Work out the finished part from the listing and answer in its coordinate system (mm). Face numbers are marked on the shaded views. A direction names the side the tool comes from. Coordinates: 2 decimals unless noted, no trailing zeros. Write each loop counter-clockwise with the first axis right and the second up, starting at its lowest first coordinate (ties: lowest second). Pieces come first, ordered by that corner, then holes. Notation, with made-up numbers: (22.5, -2.5) - (81.5, -2.5) arc R17 cw to (81.5, 26.5) - close; hole circle Ø10 at (21, 88). An arc over 180 degrees is marked (long way). One line per item, written item: value.
```python
from build123d import *

# Parameters (mm, degrees)
ESBO_O1_W                                   = 50
ESBO_O1_H                                   = 57
ESBO_O1_R                                   = 13
RESSALTO_EXTRUS_O1_DEPTH                    = 8
ESBO_O3_W                                   = 50
ESBO_O3_H                                   = 57
RESSALTO_EXTRUS_O2_DEPTH                    = 2
BROCA_DE_ROSQUEAR_PARA_TARRAXA_DE_M51_D     = 4.2
BROCA_DE_ROSQUEAR_PARA_TARRAXA_DE_M51_DEPTH = 15
BROCA_DE_ROSQUEAR_PARA_TARRAXA_DE_M51_TIP   = 1.2618073
BROCA_DE_ROSQUEAR_PARA_TARRAXA_DE_M52_D     = 4.2
BROCA_DE_ROSQUEAR_PARA_TARRAXA_DE_M52_DEPTH = 15
BROCA_DE_ROSQUEAR_PARA_TARRAXA_DE_M52_TIP   = 1.2618073


with BuildPart() as part:
    # Esboço1 → Ressalto-extrusão1 (new body)
    with BuildSketch(Plane.XY):
        with Locations((25, 28.5)):
            Rectangle(ESBO_O1_W, ESBO_O1_H)
        with Locations((25, 25)):
            Circle(ESBO_O1_R, mode=Mode.SUBTRACT)
    extrude(amount=RESSALTO_EXTRUS_O1_DEPTH)

    # Esboço3 → Ressalto-extrusão2 (add)
    with BuildSketch(Plane.XY.offset(8)):
        with Locations((25, 28.5)):
            Rectangle(ESBO_O3_W, ESBO_O3_H)
    extrude(amount=RESSALTO_EXTRUS_O2_DEPTH)

    # Broca de rosquear para tarraxa de M51
    with Locations(Plane(origin=(0, 0, 0), x_dir=(-1, 0, 0), z_dir=(0, -1, 0))):
        with Locations((-6, -5), (-44, -5)):
            Hole(BROCA_DE_ROSQUEAR_PARA_TARRAXA_DE_M51_D / 2, depth=BROCA_DE_ROSQUEAR_PARA_TARRAXA_DE_M51_DEPTH)
            with Locations((0, 0, -(BROCA_DE_ROSQUEAR_PARA_TARRAXA_DE_M51_DEPTH + BROCA_DE_ROSQUEAR_PARA_TARRAXA_DE_M51_TIP / 2))):  # 118° drill point
                Cone(0, BROCA_DE_ROSQUEAR_PARA_TARRAXA_DE_M51_D / 2, BROCA_DE_ROSQUEAR_PARA_TARRAXA_DE_M51_TIP, mode=Mode.SUBTRACT)

    # Broca de rosquear para tarraxa de M52
    with Locations(Plane(origin=(0, 57, 0), x_dir=(1, 0, 0), z_dir=(0, 1, 0))):
        with Locations((6, -5), (44, -5)):
            Hole(BROCA_DE_ROSQUEAR_PARA_TARRAXA_DE_M52_D / 2, depth=BROCA_DE_ROSQUEAR_PARA_TARRAXA_DE_M52_DEPTH)
            with Locations((0, 0, -(BROCA_DE_ROSQUEAR_PARA_TARRAXA_DE_M52_DEPTH + BROCA_DE_ROSQUEAR_PARA_TARRAXA_DE_M52_TIP / 2))):  # 118° drill point
                Cone(0, BROCA_DE_ROSQUEAR_PARA_TARRAXA_DE_M52_D / 2, BROCA_DE_ROSQUEAR_PARA_TARRAXA_DE_M52_TIP, mode=Mode.SUBTRACT)


solid = part.part
```
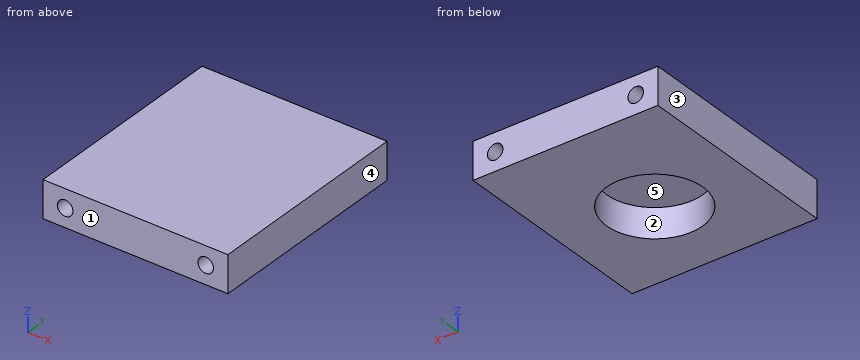
Item 1: Determine the mould class of the marked faces 1, 2 and 3 for opening direction Y: +Y half, -Y half, draft (parallel to the pull), parting line (faces both ways), or undercut.
Evaluation:
face 1: -Y half
face 2: undercut
face 3: draft
Item 2: Section D-D, the plane y = 25 is taken. Determine the outline of the cut face in (x, z), then the cut area to 3 significant figures.
Evaluation:
outline: (0, 0) - (12, 0) - (12, 8) - (38, 8) - (38, 0) - (50, 0) - (50, 10) - (0, 10) - close
area: 292 mm2
Item 3: Section B-B, the plane x = 25 is taken. Determine the outline of the cut face in (y, z).
Evaluation:
outline: (0, 0) - (12, 0) - (12, 8) - (38, 8) - (38, 0) - (57, 0) - (57, 10) - (0, 10) - close
Item 4: Given pin 1 (2.5 mm diameter, centred on x = 6, z = 5, fed in from -Y); pin 2 (4 mm diameter, centred on x = 44, z = 5, fed in from -Y); pin 3 (13 mm diameter, centred on x = 22.5, y = 26, fed in from -Z), each flat-ended and moving along its own axis, determine where each tip first touches the part or whether it passes through.
Evaluation:
pin 1: stops at y = 15.51
pin 2: stops at y = 15.06
pin 3: stops at z = 8
Item 5: Section A-A, the plane z = 1.25 is taken. Determine the outline of the cut face in (x, y).
Evaluation:
outline: (0, 0) - (50, 0) - (50, 57) - (0, 57) - close; hole circle Ø26 at (25, 25)
Item 6: Section C-C, the plane y = 11 is taken. Determine the outline of the cut face in (x, z).
Evaluation:
outline: (0, 0) - (50, 0) - (50, 10) - (0, 10) - close; hole circle Ø4.2 at (6, 5); hole circle Ø4.2 at (44, 5)
Item 7: Consider probe 1 along Z at (x, y) = (44, 7); probe 2 along Y at (x, z) = (25, 5); probe 3 along Y at (x, z) = (27, 1.75). Determine where each line is inside the solid, lowest interval first.
Evaluation:
probe 1: z = 0 to 2.9, 7.1 to 10
probe 2: y = 0 to 12, 38 to 57
probe 3: y = 0 to 12.15, 37.85 to 57
Item 8: Which of the six approach directions +Z, -Z, +X, -X, +Y, -Y give full straight-line access (tool end or side, diameter ignored) to the marked faces 4 and 5?
Evaluation:
face 4: +Z, -Z, +X, +Y, -Y
face 5: -Z
